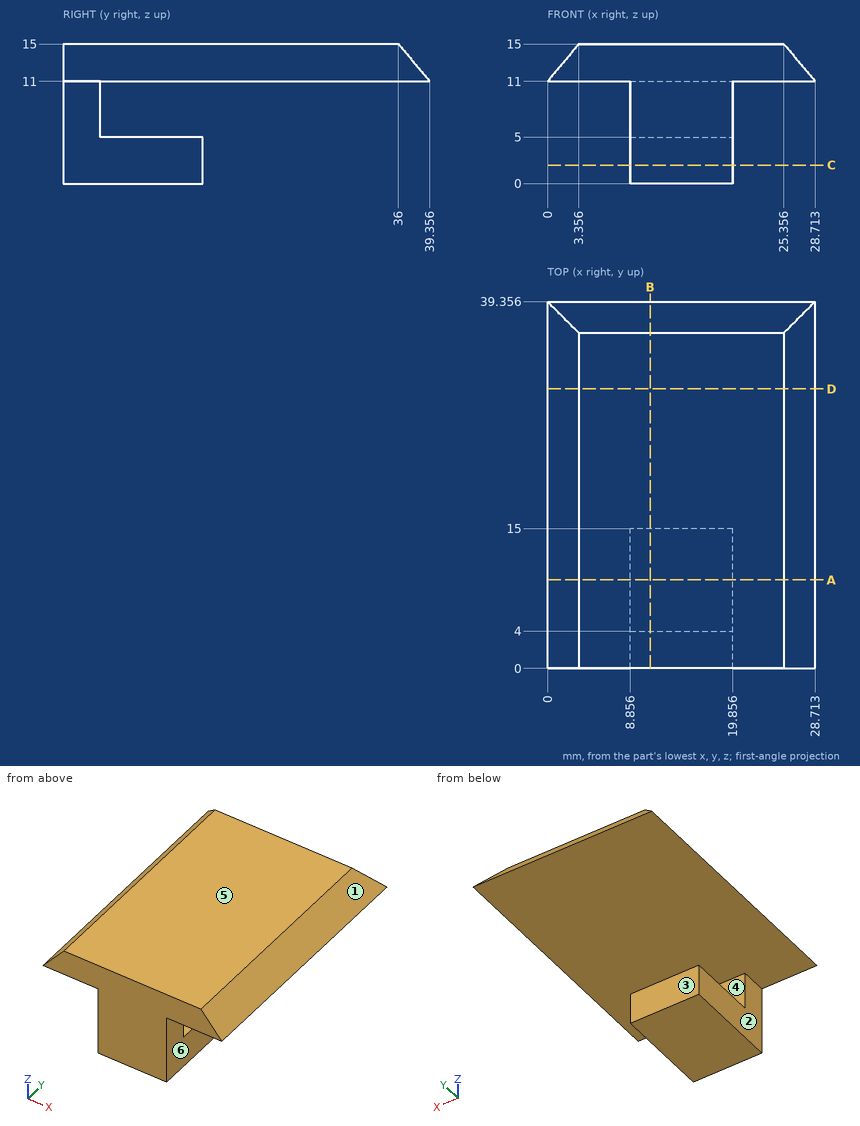
Design review of the part shown in the three views and the two pictorial views. Dimensions are in mm from the part's minimum x, y and z. A direction names the side the tool comes from. Coordinates: 2 decimals unless noted, no trailing zeros. Order: outer loops, then holes, each group sorted by start corner. A loop starts at its lowest first (then second) coordinate and runs counter-clockwise, first axis right, second up. Notation, with made-up numbers: (80.25, 50) -> (120.25, 50) arc R29 ccw to (120.25, 87) -> close; hole circle Ø5 at (41.25, 1). An arc over 180 degrees is marked (long way). Use one line per item in the form item = value. Start each with the question number.
(1) Add section C-C on z = 2. State the section outline as (x, y) points.
(2) Add section B-B on x = 11. State the section outline as (y, z) points.
(3) The part is to be moulded in two halves that separate along Z. For the marked faces 4, 5 and 6, say which applies: +Z half, -Z half, draft (parallel to the pull), parting line (faces both ways), or undercut.
(4) Add section D-D on y = 30. State the section outline as (x, z) points.
(5) For the marked faces 1, 2 and 3, list the 3-axis set-ups (+Z, -Z, +X, -X, +Y, -Y) from which the entire face can be reached by the end or side of a thin tool; tool diameter is ignored.
(6) Add section A-A on y = 9.5. State the section outline as (x, z) points.
(7) Insertion check: pin 1 (4 mm diameter, centred on x = 16, z = 2, fed in from +Y); pin 2 (1 mm diameter, centred on x = 24.5, y = 12.5, fed in from -Z); pin 3 (5.5 mm diameter, centred on y = 7.5, z = 7.5, fed in from -X). Each pin has a flat end and moves straight along its axis. Give the tip position at first contact, or say it passes through.
(8) For probe 1 along Z at (x, y) = (18, 13); probe 2 along Z at (x, y) = (22, 7); probe 3 along Y at (x, z) = (9.25, 2), list the stretches that pass through material, from the lowest coordinate up.
Answer block:
q1.outline = (8.86, 0) -> (19.86, 0) -> (19.86, 15) -> (8.86, 15) -> close
q2.outline = (0, 0) -> (15, 0) -> (15, 5) -> (4, 5) -> (4, 11) -> (39.36, 11) -> (36, 15) -> (0, 15) -> close
q3.face_4 = undercut
q3.face_5 = +Z half
q3.face_6 = draft
q4.outline = (0, 11) -> (28.71, 11) -> (25.36, 15) -> (3.36, 15) -> close
q5.face_1 = +Z, +X, +Y, -Y
q5.face_2 = -Z, -X, +Y, -Y
q5.face_3 = -Z, +X, -X, +Y
q6.outline = (0, 11) -> (28.71, 11) -> (25.36, 15) -> (3.36, 15) -> close; (8.86, 0) -> (19.86, 0) -> (19.86, 5) -> (8.86, 5) -> close
q7.pin_1 = 15
q7.pin_2 = 11
q7.pin_3 = 8.86
q8.probe_1 = 0 to 5, 11 to 15
q8.probe_2 = 11 to 15
q8.probe_3 = 0 to 15
